Input: part model. Units: mm. Frame: model coordinates. Face numbers are marked on the shaded views. Round coordinates to 2 decimals unless told otherwise and drop trailing zeros. Loops run counter-clockwise (first coordinate to the right, second up) from the corner with the lowest first, then second, coordinate; pieces in that order, holes last.
(1) Line query: line 1 (Y direction, x = 6.35, z = 2) (3 decimals); line 2 (Y direction, x = 8, z = 2.75); line 3 (Y direction, x = 2, z = 9.5). Output: solid intervals per line, ascending.
(2) Cut plane B-B, the plane y = -3.81. Output: boundary loops of the cut face in (x, z) (3 decimals), and give its area (3 significant figures).
(3) First-contact query: pin 1 Ø1.9 at (x, y) = (6, -4) entering from -Z; pin 2 Ø6 at (x, z) = (2.5, 5) entering from -Y. Flat tips, straight axial feed; report the tip coordinate or a pass-through.
(4) Cut plane C-C, the plane z = 1.25. Output: boundary loops of the cut face in (x, y) (3 decimals).
(5) Draft query along X for the marked faces 1, 2 and 3. Return one class per face: released by +X, released by -X, zero draft, split by the parting line, or undercut.
(6) Cut plane A-A, the plane x = 6.35. Output: boundary loops of the cut face in (y, z) (3 decimals).
(7) Cut plane D-D, the plane z = 9. Output: boundary loops of the cut face in (x, y), and give its area (3 significant figures).
Autodesk Inventor part; units mm, degrees
ref_plane "YZ Plane" through (0, 0, 0) normal (1, 0, 0) x (0, 1, 0)
ref_plane "XZ Plane" through (0, 0, 0) normal (0, 1, 0) x (-1, 0, 0)
ref_plane "XY Plane" through (0, 0, 0) normal (0, 0, 1) x (1, 0, 0)
sketch "Sketch1" plane through (0, 0, 0) normal (0, 0, 1) x (1, 0, 0)
  line L0 (0, 0) -> (12.7, 0)
  line L1 (12.7, 0) -> (12.7, -25.4)
  line L2 (12.7, -25.4) -> (0, -25.4)
  line L3 (0, -25.4) -> (0, 0)
  dimension "d0" = 25.4
  dimension "d1" = 12.7
extrude "Extrusion1" add sketch "Sketch1" along normal blind 12.7
sketch "Sketch2" plane through (0, 0, 12.7) normal (0, 0, 1) x (1, 0, 0)
  line L0 (0, -25.4) -> (12.7, -25.4)
  arc A0 (0, -25.4) -> (12.7, -25.4) centre (6.35, -25.3838) ccw
  point P0 (0, 0)
extrude "Extrusion2" add sketch "Sketch2" against normal blind 12.7
sketch "Sketch3" plane through (0, 0, 0) normal (0, 0, -1) x (-1, 0, 0)
  line L0 (-12.7, 0) -> (0, 0) construction
  line L1 (-6.35, 0) -> (-6.35, -3.81) construction
  circle A0 centre (-6.35, -3.81) radius 1.905
  dimension "d7" = 3.81
  dimension "d8" = 3.81
extrude "Extrusion3" cut sketch "Sketch3" against normal blind 6.35
properties part number "Finger"
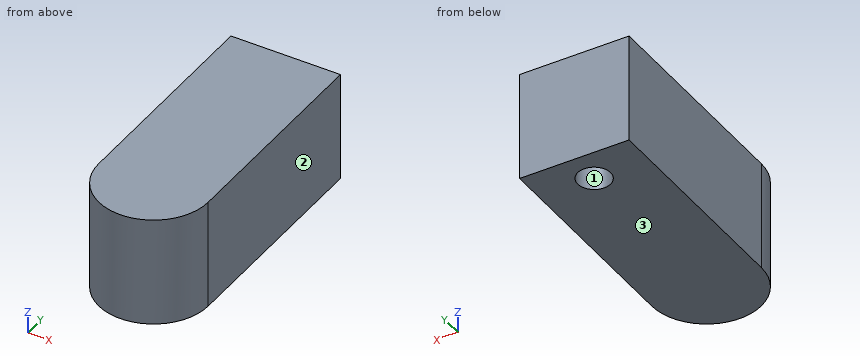
Reported:
1. line 1: y = -31.734 to -5.715, -1.905 to 0
1. line 2: y = -31.52 to -4.76, -2.86 to 0
1. line 3: y = -30.01 to 0
2. outline: (0, 0) - (4.445, 0) - (4.445, 6.35) - (8.255, 6.35) - (8.255, 0) - (12.7, 0) - (12.7, 12.7) - (0, 12.7) - close
2. area: 137 mm2
3. pin 1: stops at z = 6.35
3. pin 2: stops at y = -31.68
4. outline: (0, -25.4) arc R6.35 ccw to (12.7, -25.4) - (12.7, 0) - (0, 0) - close; hole circle Ø3.81 at (6.35, -3.81)
5. face 1: undercut
5. face 2: released by +X
5. face 3: zero draft
6. outline: (-31.734, 0) - (-5.715, 0) - (-5.715, 6.35) - (-1.905, 6.35) - (-1.905, 0) - (0, 0) - (0, 12.7) - (-31.734, 12.7) - close
7. outline: (0, -25.4) arc R6.35 ccw to (12.7, -25.4) - (12.7, 0) - (0, 0) - close
7. area: 386 mm2
